Answer from the drawing. Dimensions are ordinates in mm from the lowest x, y and z of the part. A direction names the side the tool comes from. Coordinates: 2 decimals unless noted, no trailing zeros. Order: outer loops, then holes, each group sorted by start corner. A loop starts at its lowest first (then second) coordinate and runs counter-clockwise, first axis right, second up. Notation, with made-up numbers: M 22,25.25 L 81,25.25 A10 cw 81,44.25 Z; hole C 70,-27 d3. An arc over 180 degrees is marked long. Use a Markdown table: item, result.
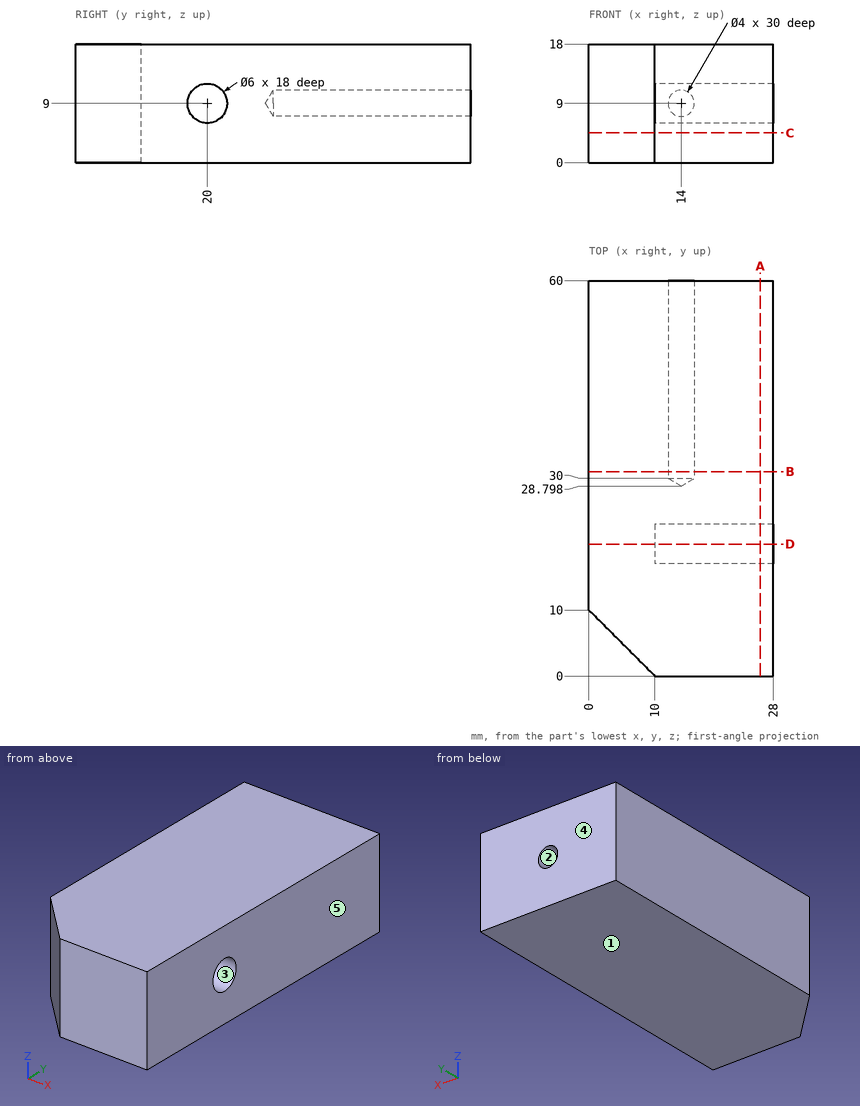
(1) A cutting plane is placed at D-D (y = 20). Determine the outline of the cut face in (x, z).
Conclusion:
| item | result |
|---|---|
| outline | M 0,0 L 28,0 L 28,6 L 10,6 L 10,12 L 28,12 L 28,18 L 0,18 Z |
(2) Determine the mould class of the marked faces 3, 4 and 5 for opening direction Y: pulls with the +Y half, pulls with the -Y half, needs draft (parallel to the pull), parting line crosses it, or undercut.
Conclusion:
| item | result |
|---|---|
| face 3 | undercut |
| face 4 | pulls with the +Y half |
| face 5 | needs draft |
(3) Given P1, Ø3, axis at y = 20, z = 10, coming from the +X side; P2, Ø1, axis at y = 16.5, z = 15, coming from the -X side, each flat-ended and moving along its own axis, determine where each tip first touches the part or whether it passes through.
Conclusion:
| item | result |
|---|---|
| P1 | x = 10 |
| P2 | x = 0 |
(4) A cutting plane is placed at B-B (y = 31). Determine the outline of the cut face in (x, z).
Conclusion:
| item | result |
|---|---|
| outline | M 0,0 L 28,0 L 28,18 L 0,18 Z; hole C 14,9 d4 |
(5) Which of the six approach directions +Z, -Z, +X, -X, +Y, -Y give full straight-line access (tool end or side, diameter ignored) to the marked faces 1 and 2?
Conclusion:
| item | result |
|---|---|
| face 1 | -Z, +X, -X, +Y, -Y |
| face 2 | +Y |
(6) Straight lines are drawn through the part: L1, parallel to X at y = 37.5, z = 9; L2, parallel to Z at x = 14, y = 48; L3, parallel to Y at x = 19.25, z = 11.75. For each, find the intervals that lie inside material, in ascending order.
Conclusion:
| item | result |
|---|---|
| L1 | 0 to 12, 16 to 28 |
| L2 | 0 to 7, 11 to 18 |
| L3 | 0 to 18.8, 21.2 to 60 |
(7) A cutting plane is placed at A-A (x = 26). Determine the outline of the cut face in (y, z), then the cut area to 3 significant figures.
Conclusion:
| item | result |
|---|---|
| outline | M 0,0 L 60,0 L 60,18 L 0,18 Z; hole C 20,9 d6 |
| area | 1,050 mm2 |
(8) A cutting plane is placed at C-C (z = 4.5). Determine the outline of the cut face in (x, y).
Conclusion:
| item | result |
|---|---|
| outline | M 0,10 L 10,0 L 28,0 L 28,60 L 0,60 Z |
